from build123d import *


with BuildPart() as part:
    # Ball socket turned profile → Turned socket body (revolve)
    with BuildSketch(Plane(origin=(0, -6.839373114, 16.171317762), x_dir=(-1, 0, 0), z_dir=(0, 0.3895270342980127, -0.9210150322068553)), mode=Mode.PRIVATE) as turned_socket_body_sk:
        with BuildLine():
            Line((21.450363513, -86.228362345), (21.288694752, -84.679417142))
            Line((21.288694752, -84.679417142), (22.034642647, -84.601559983))
            Line((22.034642647, -84.601559983), (22.283785554, -86.988593249))
            Line((22.283785554, -86.988593249), (23.02973345, -86.91073609))
            Line((23.02973345, -86.91073609), (23.060876313, -87.209115249))
            ThreePointArc((23.060876313, -87.209115249), (20.609484536, -88.906958963), (20.724096138, -91.886700412))
            Line((20.724096138, -91.886700412), (19.804272172, -93.020911066))
            ThreePointArc((19.804272172, -93.020911066), (19.009273884, -89.232523486), (21.450363513, -86.228362345))
        make_face()
    revolve(turned_socket_body_sk.sketch.rotate(Axis((-24.42078135, -99.160389667, -22.874224953), (0.10380954475082833, 0.9160389667138149, 0.3874224953206928)), 90), axis=Axis((-24.42078135, -99.160389667, -22.874224953), (0.10380954475082833, 0.9160389667138149, 0.3874224953206928)))


with BuildPart() as body_2:
    # Mirror1: mirrored copy
    add(part.part.mirror(Plane(origin=(0, 0, 0), x_dir=(0, 0, 1), z_dir=(0, -1, 0))))


solid = body_2.part
The listing builds one solid part. Answer for the finished solid, in the listing's coordinates (mm). Round coordinates to 2 decimals unless told otherwise and drop trailing zeros. Write each loop counter-clockwise with the first axis right and the second up, starting at its lowest first coordinate (ties: lowest second). Pieces come first, ordered by that corner, then holes. Notation, with made-up numbers: M -29.75,68 L 0.25,68 A36 ccw 0.25,107 Z; hole C -23.5,-24.75 d7. An arc over 180 degrees is marked long. Write each question's results on one line, items separated by ' | '. Start each with the question number.
(1) Determine the mould class of faces 1 (the cylindrical face through (-21.95, 85.94, -15.99)), 2 (the cylindrical face through (-22.94, 86.09, -16.533)), 3 (the flat face through (-22.14, 84.5, -17.37)) for opening direction Y: +Y half, -Y half, draft (parallel to the pull), parting line (faces both ways), or undercut.
(2) The part is cut by section A-A, the plane y = 87.75. Write down the section's boundary in (x, z).
(3) Find the intervals of material crossed by line 1 (X direction, y = 90.75, z = -19.5); line 2 (X direction, y = 90, z = -17.5); line 3 (Z direction, x = -23.75, y = 88.5), in increasing order.
(4) The part is cut by section B-B, the plane z = -15. Write down the section's boundary in (x, y).
(5) This flat-tipped pin is pushed along its axis until it touches: P1, Ø2, axis at x = -26.5, y = 90.5, coming from the -Z side. Where does it stop, or does it pass through?
(6) The part is cut by section C-C, the plane x = -19.25. Write down the section's boundary in (y, z).
Worked answers:
1) face 1: undercut | face 2: undercut | face 3: -Y half
2) outline: C -23.38,-19 d7.79; hole C -23.38,-19 d4.26
3) line 1: x = -27.79 to -26.35, -20.42 to -18.97 | line 2: x = -27.63 to -26.1, -20.67 to -19.14 | line 3: z = -23.23 to -21.69, -16.31 to -14.77
4) outline: C -23.38,90 d4.12
5) P1: stops at z = -22.95
6) outline: C 90,-19 d3.56
